from build123d import *

# Parameters (mm, degrees)
BOSS_EXTRUDE1_DEPTH = 6.35
SKETCH2_R           = 3.5
CUT_EXTRUDE1_DEPTH  = 7.35


with BuildPart() as part:
    # Sketch1 → Boss-Extrude1 (new body)
    with BuildSketch(Plane.XY):
        Polygon((-25.4, 50.8), (-25.4, 76.2), (0, 127), (25.4, 127), (50.8, 76.2), (50.8, 50.8), (25.4, 0), (0, 0), align=None)
    extrude(amount=BOSS_EXTRUDE1_DEPTH)

    # Sketch2 → Cut-Extrude1 (cut, through all)
    with BuildSketch(Plane.XY.offset(6.35)):
        with Locations((12.7, 63.5)):
            Circle(SKETCH2_R)
        with Locations((38.1, 63.5)):
            Circle(SKETCH2_R)
        with Locations((-12.7, 63.5)):
            Circle(SKETCH2_R)
        with Locations((12.7, 38.1)):
            Circle(SKETCH2_R)
        with Locations((12.7, 12.7)):
            Circle(SKETCH2_R)
        with Locations((12.7, 114.3)):
            Circle(SKETCH2_R)
        with Locations((12.7, 88.9)):
            Circle(SKETCH2_R)
    extrude(amount=-CUT_EXTRUDE1_DEPTH, mode=Mode.SUBTRACT)


solid = part.part
Here's how the part is built. I have some questions about the finished solid (model axes, mm). Give positions to 0.01 mm unless a question says otherwise; leave off trailing zeros. Order: outer loops, then holes, each group sorted by start corner. A loop starts at its lowest first (then second) coordinate and runs counter-clockwise, first axis right, second up. Notation, with made-up numbers: (-18.75, -35) -> (28.25, -35) arc R25 cw to (28.25, -8) -> close; hole circle Ø3 at (84.25, -9.75). An arc over 180 degrees is marked (long way). One line per item, written item: value. Start each with the question number.
1. Imagine slicing it at B-B, the plane y = 12.7. List the corners of the cut face in (x, z) for me, plus the area to 3 significant figures.
2. Imagine slicing it at D-D, the plane z = 2.75. List the corners of the cut face in (x, y) for me, plus the area to 3 significant figures.
3. I need wall thicknesses on probe 1 along Y at (x, z) = (12.7, 2); probe 2 along Y at (x, z) = (12, 3.25); probe 3 along Y at (x, z) = (-12, 2). Which ranges of each line are inside material? Lowest first, please. Write a range as from..to.
4. Imagine slicing it at C-C, the plane y = 63.5. List the corners of the cut face in (x, z) for me, plus the area to 3 significant figures.
5. Will these pins go through, and if not, where does the flat tip stop? pin 1 Ø4 at (x, y) = (12.7, 38.1) entering from -Z; pin 2 Ø1 at (x, z) = (0, 5) entering from -Y; pin 3 Ø3 at (y, z) = (82, 4) entering from +X.
6. We'd pull the mould along Y, two halves only. Please class faces 1 (the face through (-13, 101, 3)), 2 (the face through (12.24, 117.77, 3.22)), 3 (the face through (50.8, 64, 3)): released by +Y, released by -Y, zero draft, split by the parting line, or undercut.
7. Imagine slicing it at A-A, the plane x = 38.1. List the corners of the cut face in (y, z) for me.
Values follow:
1. outline: (-6.35, 0) -> (9.2, 0) -> (9.2, 6.35) -> (-6.35, 6.35) -> close; (16.2, 0) -> (31.75, 0) -> (31.75, 6.35) -> (16.2, 6.35) -> close
1. area: 197 mm2
2. outline: (-25.4, 50.8) -> (0, 0) -> (25.4, 0) -> (50.8, 50.8) -> (50.8, 76.2) -> (25.4, 127) -> (0, 127) -> (-25.4, 76.2) -> close; hole circle Ø7 at (-12.7, 63.5); hole circle Ø7 at (12.7, 12.7); hole circle Ø7 at (12.7, 38.1); hole circle Ø7 at (12.7, 63.5); hole circle Ø7 at (12.7, 88.9); hole circle Ø7 at (12.7, 114.3); hole circle Ø7 at (38.1, 63.5)
2. area: 6,830 mm2
3. probe 1: y = 0..9.2, 16.2..34.6, 41.6..60, 67..85.4, 92.4..110.8, 117.8..127
3. probe 2: y = 0..9.27, 16.13..34.67, 41.53..60.07, 66.93..85.47, 92.33..110.87, 117.73..127
3. probe 3: y = 24..60.07, 66.93..103
4. outline: (-25.4, 0) -> (-16.2, 0) -> (-16.2, 6.35) -> (-25.4, 6.35) -> close; (-9.2, 0) -> (9.2, 0) -> (9.2, 6.35) -> (-9.2, 6.35) -> close; (16.2, 0) -> (34.6, 0) -> (34.6, 6.35) -> (16.2, 6.35) -> close; (41.6, 0) -> (50.8, 0) -> (50.8, 6.35) -> (41.6, 6.35) -> close
4. area: 351 mm2
5. pin 1: passes through
5. pin 2: stops at y = 0
5. pin 3: stops at x = 48.65
6. face 1: released by +Y
6. face 2: undercut
6. face 3: zero draft
7. outline: (25.4, 0) -> (60, 0) -> (60, 6.35) -> (25.4, 6.35) -> close; (67, 0) -> (101.6, 0) -> (101.6, 6.35) -> (67, 6.35) -> close
